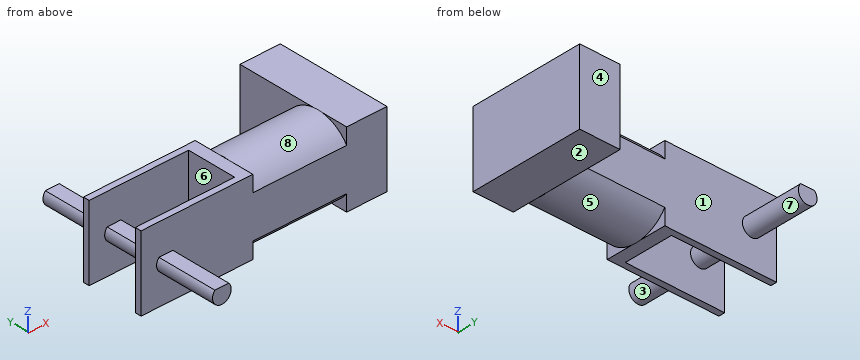
```python
from build123d import *

# Parameters (mm, degrees)
PAD_DEPTH    = 6
PAD001_DEPTH = 14.7
PAD002_DEPTH = 15.1
SKETCH003_W  = 18.5
SKETCH003_H  = 12
PAD003_DEPTH = 6.5


with BuildPart() as part:
    # Sketch → Pad (new body, symmetric)
    with BuildSketch(Plane.XY):
        Polygon((-4, 5), (14, 5), (14, -5), (-4, -5), (-4, -4), (12, -4), (12, 4), (-4, 4), align=None)
    extrude(amount=PAD_DEPTH, both=True)

    # Sketch001 → Pad001 (join, symmetric)
    with BuildSketch(Plane.XZ):
        with BuildLine():
            ThreePointArc((-1.118034, 1), (0, -1.5), (1.118034, 1))
            Line((-1.118034, 1), (1.118034, 1))
        make_face()
    extrude(amount=PAD001_DEPTH, both=True)

    # Sketch002 (on DatumPlane) → Pad002 (join)
    with BuildSketch(Plane.YZ.offset(14)):
        with BuildLine():
            ThreePointArc((5, 3.406244), (0, 6.05), (-5, 3.406244))
            Line((-5, -3.406244), (-5, 3.406244))
            ThreePointArc((-5, -3.406244), (0, -6.05), (5, -3.406244))
            Line((5, 3.406244), (5, -3.406244))
        make_face()
    extrude(amount=PAD002_DEPTH)

    # Sketch003 (on DatumPlane) → Pad003 (join)
    with BuildSketch(Plane.YZ.offset(29.1)):
        with Locations((4.25, 0)):
            Rectangle(SKETCH003_W, SKETCH003_H)
    extrude(amount=PAD003_DEPTH)


solid = part.part
```
Geometry: final body of the model. Coordinates: model frame, mm. Face numbers are marked on the shaded views. A direction names the side the tool comes from. Round coordinates to 2 decimals unless told otherwise and drop trailing zeros. Loops run counter-clockwise (first coordinate to the right, second up) from the corner with the lowest first, then second, coordinate; pieces in that order, holes last. Notation, with made-up numbers: (-29.5, 33.25) -> (14.5, 33.25) arc R17 cw to (14.5, 54.25) -> close; hole circle Ø6 at (-25, 47.25). An arc over 180 degrees is marked (long way). Use one line per item in the form item = value.
Item 1: Cut plane B-B on x = 9.5. Output: boundary loops of the cut face in (y, z), then the cut area to 3 significant figures.
Evaluation:
outline = (-5, -6) -> (-4, -6) -> (-4, 6) -> (-5, 6) -> close; (4, -6) -> (5, -6) -> (5, 6) -> (4, 6) -> close
area = 24.0 mm2
Item 2: Contact query for flat-ended pins moving along their axis: pin 1 Ø1.3 at (y, z) = (-2, -5.5) entering from -X; pin 2 Ø3.5 at (x, z) = (10, -2) entering from -Y; pin 3 Ø5 at (x, y) = (9, 0) entering from -Z; pin 4 Ø1 at (y, z) = (8.5, 2.5) entering from -X. Output: stop coordinate, or through.
Evaluation:
pin_1 = 12
pin_2 = -5
pin_3 = through
pin_4 = 29.1
Item 3: Cut plane A-A on y = 13. Output: boundary loops of the cut face in (x, z), then the cut area to 3 significant figures.
Evaluation:
outline = (-1.12, 1) arc R1.5 ccw (long way) to (1.12, 1) -> close; (29.1, -6) -> (35.6, -6) -> (35.6, 6) -> (29.1, 6) -> close
area = 84.3 mm2
Item 4: Access query for the marked faces 4, 5, 6, 7 and 8. Directions: +Z, -Z, +X, -X, +Y, -Y. A direction counts if a zero-diameter tool reaches every point of the face in a straight line with its end or side. Return the directions, or none.
Evaluation:
face_4 = +Z, -Z, +X, +Y
face_5 = -Z
face_6 = +Z, -Z
face_7 = +Y
face_8 = +Z
Item 5: Draft query along X for the marked faces 1, 2 and 3. Return one class per face: released by +X, released by -X, zero draft, split by the parting line, or undercut.
Evaluation:
face_1 = undercut
face_2 = zero draft
face_3 = split by the parting line
Item 6: Cut plane C-C on z = 0. Output: boundary loops of the cut face in (x, y).
Evaluation:
outline = (-4, -5) -> (-1.5, -5) -> (-1.5, -14.7) -> (1.5, -14.7) -> (1.5, -5) -> (35.6, -5) -> (35.6, 13.5) -> (29.1, 13.5) -> (29.1, 5) -> (1.5, 5) -> (1.5, 14.7) -> (-1.5, 14.7) -> (-1.5, 5) -> (-4, 5) -> (-4, 4) -> (-1.5, 4) -> (-1.5, -4) -> (-4, -4) -> close; hole (1.5, -4) -> (12, -4) -> (12, 4) -> (1.5, 4) -> close
Item 7: Cut plane D-D on x = 0. Output: boundary loops of the cut face in (y, z).
Evaluation:
outline = (-14.7, -1.5) -> (-5, -1.5) -> (-5, -6) -> (-4, -6) -> (-4, -1.5) -> (4, -1.5) -> (4, -6) -> (5, -6) -> (5, -1.5) -> (14.7, -1.5) -> (14.7, 1) -> (5, 1) -> (5, 6) -> (4, 6) -> (4, 1) -> (-4, 1) -> (-4, 6) -> (-5, 6) -> (-5, 1) -> (-14.7, 1) -> close
Item 8: Material intervals for probe 1 along Y at (x, z) = (10, -1.5); probe 2 along X at (y, z) = (-1, -2.5); probe 3 along Z at (x, y) = (1, 9.5), sorted ascending.
Evaluation:
probe_1 = -5 to -4, 4 to 5
probe_2 = 12 to 35.6
probe_3 = -1.12 to 1
